```python
from build123d import *

# Parameters (mm, degrees)
F0_W     = 50.8
F0_H     = 50.8
F1_DEPTH = 1219.2
F3_DEPTH = 19.05
F4_W     = 31.75
F4_H     = 31.75
F5_DEPTH = 1200.151


with BuildPart() as f1:
    # F0 (on Top) → F1 (new body)
    with BuildSketch(Plane.XY):
        with Locations((25.4, 25.4)):
            Rectangle(F0_W, F0_H)
    extrude(amount=-F1_DEPTH)

    # F2 (on face) → F3 (cut)
    with BuildSketch(Plane.XY):
        Polygon((19.05, 31.75), (0, 31.75), (0, 0), (50.8, 0), (50.8, 50.8), (19.05, 50.8), align=None)
    extrude(amount=-F3_DEPTH, mode=Mode.SUBTRACT)

    # F4 (on face) → F5 (cut, through all)
    with BuildSketch(Plane.XY.offset(-19.05)):
        with Locations((34.925, 15.875)):
            Rectangle(F4_W, F4_H)
    extrude(amount=-F5_DEPTH, mode=Mode.SUBTRACT)


solid = f1.part
```
Here's how the part is built. I have some questions about the finished solid (model axes, mm). A direction names the side the tool comes from. Coordinates: 2 decimals unless noted, no trailing zeros. Order: outer loops, then holes, each group sorted by start corner. A loop starts at its lowest first (then second) coordinate and runs counter-clockwise, first axis right, second up. Notation, with made-up numbers: (-35, 2) - (-1, 2) arc R12 cw to (-1, 13) - close; hole circle Ø4 at (5.5, 81.5). An arc over 180 degrees is marked (long way). One line per question, with ' | ' between items.
(1) Will these pins go through, and if not, where does the flat tip stop? pin 1 (4 mm diameter, centred on x = 29, z = -1066, fed in from -Y); pin 2 (4 mm diameter, centred on x = 12.5, y = 10.5, fed in from +Z); pin 3 (3 mm diameter, centred on y = 18, z = -232, fed in from +X).
Report:
pin 1: stops at y = 31.75 | pin 2: stops at z = -19.05 | pin 3: stops at x = 19.05
(2) If we mould it in two halves opening along Z, with no side actions, what happens to faces 6 (the flat face through (19.05, 16, -611)), 7 (the flat face through (35, 41, -19.05)), 8 (the flat face through (19, 37, -1219.2))? For each: pulls with the +Z half, pulls with the -Z half, needs draft (parallel to the pull), parting line crosses it, or undercut.
Report:
face 6: needs draft | face 7: pulls with the +Z half | face 8: pulls with the -Z half
(3) Suppose I cut it at C-C on y = 23. List the corners of the cut face in (x, z) for me, and give its area (3 significant figures).
Report:
outline: (0, -1219.2) - (19.05, -1219.2) - (19.05, -19.05) - (0, -19.05) - close | area: 22,900 mm2
(4) Suppose I cut it at B-B on x = 42. List the corners of the cut face in (y, z) for me.
Report:
outline: (31.75, -1219.2) - (50.8, -1219.2) - (50.8, -19.05) - (31.75, -19.05) - close
(5) If I drill on L1, parallel to Y at x = 34.5, z = -53; L2, parallel to X at y = 24.5, z = -302.5; L3, parallel to Z at x = 11, y = 20, over which ranges is the centre line in solid material (lowest first)?
Report:
L1: y = 31.75 to 50.8 | L2: x = 0 to 19.05 | L3: z = -1219.2 to -19.05
(6) For faces 1 (the flat face through (9, 0, -611)), 2 (the flat face through (9, 16, -19.05)), 3 (the flat face through (9, 41, 0)), 4 (the flat face through (35, 31.75, -611)), 5 (the flat face through (19.05, 41, -9)), which set-ups out of +Z, -Z, +X, -X, +Y, -Y let a thin tool reach every point of the face, with its end or its side?
Report:
face 1: +Z, -Z, +X, -X, -Y | face 2: +Z, +X, -X, -Y | face 3: +Z, +X, -X, +Y, -Y | face 4: +Z, -Z, +X, -Y | face 5: +Z, +X, +Y, -Y
(7) Suppose I cut it at A-A on z = -820. List the corners of the cut face in (x, y) for me, and give its area (3 significant figures).
Report:
outline: (0, 0) - (19.05, 0) - (19.05, 31.75) - (50.8, 31.75) - (50.8, 50.8) - (0, 50.8) - close | area: 1,570 mm2
